Print and shaded views of the part. All mm, measured from the part's lowest x, y and z. Give positions to 0.01 mm unless a question says otherwise; leave off trailing zeros. Write each loop counter-clockwise with the first axis right and the second up, starting at its lowest first coordinate (ties: lowest second). Pieces come first, ordered by that corner, then holes. Notation, with made-up numbers: (2, 63.25) -> (31, 63.25) arc R16 cw to (31, 93.25) -> close; hole circle Ø11 at (50.25, 66). An arc over 180 degrees is marked (long way). Put each result on its own line as item: value.
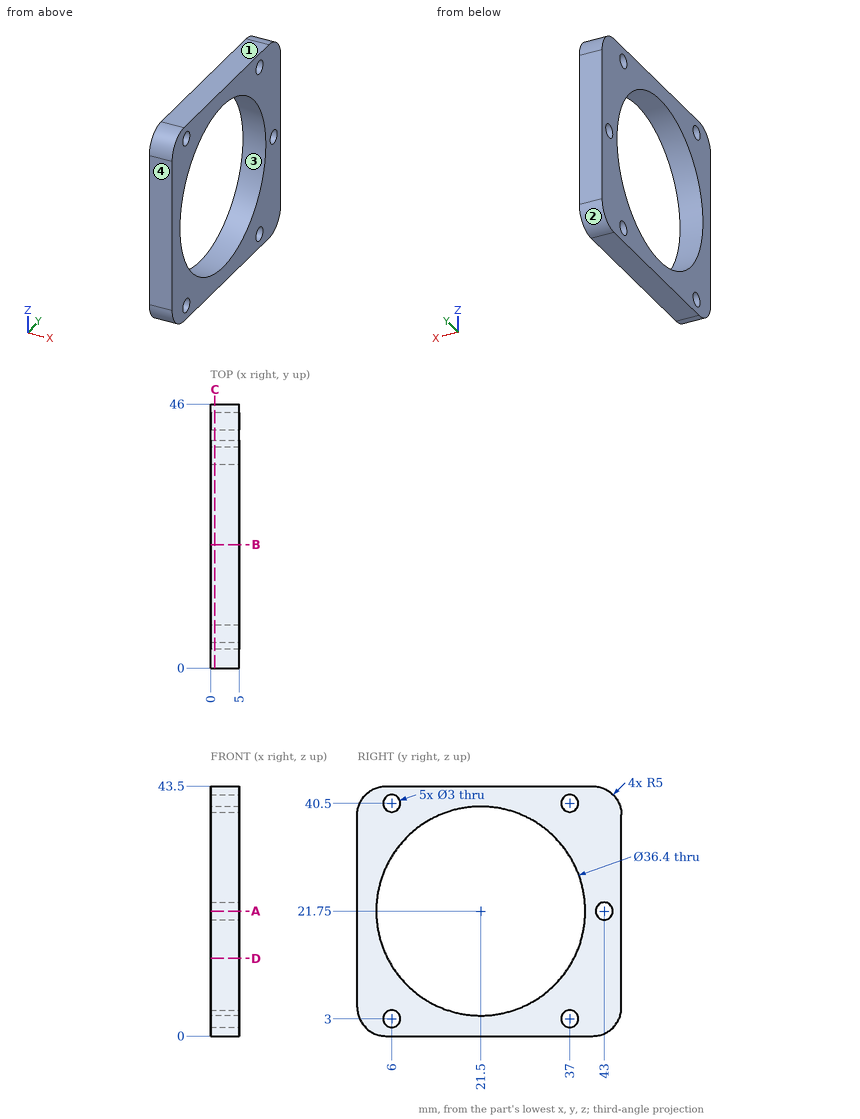
1) Slice it at D-D (z = 13.5). Write the cut outline in (x, y), plus the area to 3 significant figures.
Filled sheet:
outline: (0, 0) -> (5, 0) -> (5, 5.28) -> (0, 5.28) -> close; (0, 37.72) -> (5, 37.72) -> (5, 46) -> (0, 46) -> close
area: 67.8 mm2
2) Slice it at C-C (x = 0.75). Write the cut outline in (y, z), plus the area to 3 significant figures.
Filled sheet:
outline: (0, 5) arc R5 ccw to (5, 0) -> (41, 0) arc R5 ccw to (46, 5) -> (46, 38.5) arc R5 ccw to (41, 43.5) -> (5, 43.5) arc R5 ccw to (0, 38.5) -> close; hole circle Ø36.4 at (21.5, 21.75); hole circle Ø3 at (6, 3); hole circle Ø3 at (6, 40.5); hole circle Ø3 at (37, 3); hole circle Ø3 at (37, 40.5); hole circle Ø3 at (43, 21.75)
area: 904 mm2
3) Slice it at A-A (z = 21.75). Write the cut outline in (x, y).
Filled sheet:
outline: (0, 0) -> (5, 0) -> (5, 3.3) -> (0, 3.3) -> close; (0, 39.7) -> (5, 39.7) -> (5, 41.5) -> (0, 41.5) -> close; (0, 44.5) -> (5, 44.5) -> (5, 46) -> (0, 46) -> close
4) Wall check: L1, parallel to Z at x = 1.3, y = 7; L2, parallel to Z at x = 3.95, y = 6; L3, parallel to Z at x = 3.6, y = 21. Give the ranges that are in metal, low to high.
Filled sheet:
L1: 0 to 1.88, 4.12 to 10.75, 32.75 to 39.38, 41.62 to 43.5
L2: 0 to 1.5, 4.5 to 12.21, 31.29 to 39, 42 to 43.5
L3: 0 to 3.56, 39.94 to 43.5
5) Slice it at B-B (y = 21.5). Write the cut outline in (x, z).
Filled sheet:
outline: (0, 0) -> (5, 0) -> (5, 3.55) -> (0, 3.55) -> close; (0, 39.95) -> (5, 39.95) -> (5, 43.5) -> (0, 43.5) -> close
6) Pin check, flat tip, straight feed: pin 1 (2.5 mm diameter, centred on y = 37, z = 40.5, fed in from +X). Stop position of the tip, or through.
Filled sheet:
pin 1: through
7) Pull direction Y, two halves, no side cores. Call the marked faces 1, 2, 3 and 4: released by +Y, released by -Y, zero draft, split by the parting line, or undercut.
Filled sheet:
face 1: zero draft
face 2: released by +Y
face 3: undercut
face 4: released by -Y
